from build123d import *

# Parameters (mm, degrees)
SKETCH1_R                                       = 45
SKETCH1_R_2                                     = 2
EXTRUDE1_DEPTH                                  = 5
SKETCH2_R                                       = 28
EXTRUDE2_DEPTH                                  = 13
SKETCH3_R                                       = 25
EXTRUDE3_DEPTH                                  = 150.7
SKETCH4_R                                       = 20
CUT_EXTRUDE1_DEPTH                              = 200
CUT_EXTRUDE2_START                              = -6.2
SKETCH5_R                                       = 25
SKETCH5_R_2                                     = 22.9
CUT_EXTRUDE2_DEPTH                              = 2.2
BOSS_EXTRUDE1_START                             = 3
SKETCH6_R                                       = 25
SKETCH6_R_2                                     = 20
BOSS_EXTRUDE1_DEPTH                             = 3
CSK_FOR_M4_FLAT_HEAD_MACHINE_SCREW1_D           = 4.5
CSK_FOR_M4_FLAT_HEAD_MACHINE_SCREW1_CSINK_D     = 9.4
CSK_FOR_M4_FLAT_HEAD_MACHINE_SCREW1_CSINK_ANGLE = 90


with BuildPart() as part:
    # Sketch1 → Extrude1 (new body)
    with BuildSketch(Plane.XY):
        Circle(SKETCH1_R)
        with Locations((-34.641016151, -20)):
            Circle(SKETCH1_R_2, mode=Mode.SUBTRACT)
        with Locations((-34.641016151, 20)):
            Circle(SKETCH1_R_2, mode=Mode.SUBTRACT)
        with Locations((0, 40)):
            Circle(SKETCH1_R_2, mode=Mode.SUBTRACT)
        with Locations((0, -40)):
            Circle(SKETCH1_R_2, mode=Mode.SUBTRACT)
        with Locations((34.641016151, 20)):
            Circle(SKETCH1_R_2, mode=Mode.SUBTRACT)
        with Locations((34.641016151, -20)):
            Circle(SKETCH1_R_2, mode=Mode.SUBTRACT)
    extrude(amount=EXTRUDE1_DEPTH)

    # Sketch2 → Extrude2 (add)
    with BuildSketch(Plane.XY.offset(5)):
        with Locations(Location((0, 0, 0), (0, 0, 180))):
            Circle(SKETCH2_R)
    extrude(amount=EXTRUDE2_DEPTH)

    # Sketch3 → Extrude3 (add)
    with BuildSketch(Plane.XY.offset(18)):
        Circle(SKETCH3_R)
    extrude(amount=EXTRUDE3_DEPTH)

    # Sketch4 → Cut-Extrude1 (cut)
    with BuildSketch(Plane.XY.offset(168.7)):
        Circle(SKETCH4_R)
    extrude(amount=-CUT_EXTRUDE1_DEPTH, mode=Mode.SUBTRACT)

    # Sketch5 → Cut-Extrude2 (cut)
    with BuildSketch(Plane.XY.offset(168.7).offset(CUT_EXTRUDE2_START)):
        Circle(SKETCH5_R)
        Circle(SKETCH5_R_2, mode=Mode.SUBTRACT)
    extrude(amount=CUT_EXTRUDE2_DEPTH, mode=Mode.SUBTRACT)

    # Sketch6 → Boss-Extrude1 (add)
    with BuildSketch(Plane(origin=(0, 0, 0), x_dir=(-1, 0, 0), z_dir=(0, 0, -1)).offset(BOSS_EXTRUDE1_START)):
        with Locations(Location((0, 0, 0), (0, 0, 180))):
            Circle(SKETCH6_R)
        with Locations(Location((0, 0, 0), (0, 0, 180))):
            Circle(SKETCH6_R_2, mode=Mode.SUBTRACT)
    extrude(amount=-BOSS_EXTRUDE1_DEPTH)

    # CSK for M4 Flat Head Machine Screw1 (through all)
    with Locations(Plane.XY.offset(5)):
        with Locations((34.641016151, -20), (0, -40), (-34.641016151, -20), (-34.641016151, 20), (0, 40), (34.641016151, 20)):
            CounterSinkHole(CSK_FOR_M4_FLAT_HEAD_MACHINE_SCREW1_D / 2, CSK_FOR_M4_FLAT_HEAD_MACHINE_SCREW1_CSINK_D / 2, counter_sink_angle=CSK_FOR_M4_FLAT_HEAD_MACHINE_SCREW1_CSINK_ANGLE)


solid = part.part
Input: part model. Units: mm. Frame: model coordinates. A direction names the side the tool comes from. Round coordinates to 2 decimals unless told otherwise and drop trailing zeros. Order: outer loops, then holes, each group sorted by start corner. A loop starts at its lowest first (then second) coordinate and runs counter-clockwise, first axis right, second up.
1. Material intervals for line 1 (Y direction, x = 0, z = 1); line 2 (Z direction, x = 14, y = 29); line 3 (Y direction, x = 14.5, z = 44), sorted ascending.
The answers:
line 1: y = -45 to -42.25, -37.75 to -20, 20 to 37.75, 42.25 to 45
line 2: z = 0 to 5
line 3: y = -20.37 to -13.77, 13.77 to 20.37
2. Cut plane B-B, the plane x = -11. Output: boundary loops of the cut face in (y, z).
The answers:
outline: (-43.63, 0) - (-22.45, 0) - (-22.45, -3) - (-16.7, -3) - (-16.7, 168.7) - (-22.45, 168.7) - (-22.45, 164.7) - (-20.09, 164.7) - (-20.09, 162.5) - (-22.45, 162.5) - (-22.45, 18) - (-25.75, 18) - (-25.75, 5) - (-43.63, 5) - close; (16.7, -3) - (22.45, -3) - (22.45, 0) - (43.63, 0) - (43.63, 5) - (25.75, 5) - (25.75, 18) - (22.45, 18) - (22.45, 162.5) - (20.09, 162.5) - (20.09, 164.7) - (22.45, 164.7) - (22.45, 168.7) - (16.7, 168.7) - close
3. Set-up query: faces 5 (the face through (11, -20.3, 164.7)), 6 (the face through (23.846, 7.509, 89.238)), 7 (the face through (19, -19, 0)). Return all of +Z, -Z, +X, -X, +Y, -Y with unobstructed straight access to the full face (end or side cutting, diameter ignored); none if empty.
The answers:
face 5: none
face 6: +Z
face 7: -Z
4. Pin query (flat end, axial travel): P1, Ø12, axis at y = -5, z = 105.5, coming from the +X side; P2, Ø6, axis at x = 34.64, y = 20, coming from the -Z side; P3, Ø7, axis at x = -34.64, y = -20, coming from the +Z side. Return the tip coordinate at first contact, or that it passes through.
The answers:
P1: stops at x = 25
P2: stops at z = 0
P3: stops at z = 3.8
5. Cut plane D-D, the plane z = 92.5. Output: boundary loops of the cut face in (x, y).
The answers:
outline: circle Ø50 at (0, 0); hole circle Ø40 at (0, 0)
6. Cut plane C-C, the plane x = 0. State how many separate pieces and enclosed holes the cut face has, then the cut area to 3 significant figures.
The answers:
separate pieces: 4
enclosed holes: 0
area: 1,930 mm2
7. Mould query, pull axis Z, two halves, no side actions, for faces 1 (the face through (-35.679, -21.996, 1.257)), 2 (the face through (11, -20.3, 162.5)), 3 (the face through (-4.964, -22.355, 163.585)), 4 (the face through (33.548, 17.898, 2.669)). Classes: released by +Z, released by -Z, zero draft, split by the parting line, or undercut.
The answers:
face 1: zero draft
face 2: undercut
face 3: undercut
face 4: released by +Z
8. Cut plane A-A, the plane y = 0. Output: boundary loops of the cut face in (x, z), then the cut area to 3 significant figures.
The answers:
outline: (-45, 0) - (-25, 0) - (-25, -3) - (-20, -3) - (-20, 168.7) - (-25, 168.7) - (-25, 164.7) - (-22.9, 164.7) - (-22.9, 162.5) - (-25, 162.5) - (-25, 18) - (-28, 18) - (-28, 5) - (-45, 5) - close; (20, -3) - (25, -3) - (25, 0) - (45, 0) - (45, 5) - (28, 5) - (28, 18) - (25, 18) - (25, 162.5) - (22.9, 162.5) - (22.9, 164.7) - (25, 164.7) - (25, 168.7) - (20, 168.7) - close
area: 1,990 mm2
